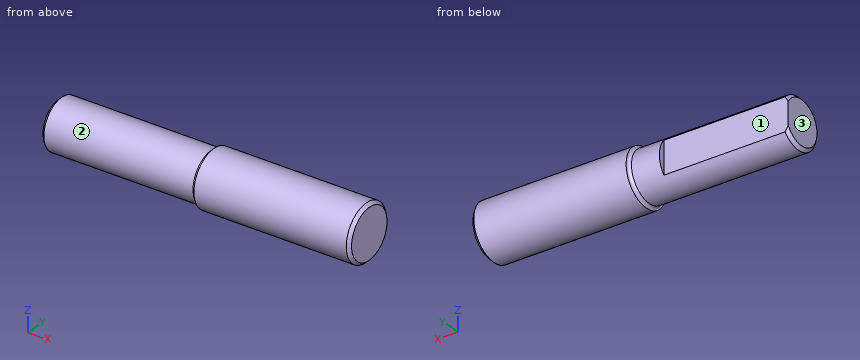
from build123d import *

# Parameters (mm, degrees)
CUT_EXTRUDE_1_DEPTH = 20


with BuildPart() as part:
    # 草图1 → 旋转1 (revolve)
    with BuildSketch(Plane.XY, mode=Mode.PRIVATE) as revolve_1_sk:
        with BuildLine():
            Line((25, 0), (25, 4))
            Line((25, 4), (24.5, 4.5))
            Line((24.5, 4.5), (0, 4.5))
            ThreePointArc((0, 4.5), (-0.146446609, 4.146446609), (-0.5, 4))
            Line((-0.5, 4), (-24.5, 4))
            Line((-24.5, 4), (-25, 3.5))
            Line((-25, 3.5), (-25, 0))
            Line((-25, 0), (25, 0))
        make_face()
    revolve(revolve_1_sk.sketch.rotate(Axis((-25, 0, 0), (1, 0, 0)), 180), axis=Axis((-25, 0, 0), (1, 0, 0)))

    # 草图2 → 切除-拉伸1 (cut)
    with BuildSketch(Plane.ZY.offset(25)):
        with BuildLine():
            Line((-2.645751311, 3), (2.645751311, 3))
            ThreePointArc((2.645751311, 3), (0, 4), (-2.645751311, 3))
        make_face()
    extrude(amount=-CUT_EXTRUDE_1_DEPTH, mode=Mode.SUBTRACT)


solid = part.part
Verification items for the finished model (mm, model axes). Face numbers are marked on the shaded views. A direction names the side the tool comes from. Give positions to 0.01 mm unless a question says otherwise; leave off trailing zeros. Loops run counter-clockwise (first coordinate to the right, second up) from the corner with the lowest first, then second, coordinate; pieces in that order, holes last.
1) Depth check by flat-ended pin: pin 1 Ø1 at (x, y) = (18, 1) entering from -Z; pin 2 Ø1 at (x, z) = (19, -2) entering from -Y. Enter the tip coordinate at first touch or a pass-through.
2) Sectioned sample at B-B, the plane y = 0. Enter the section's corners in (x, z).
3) Set-up check for the marked faces 1, 2 and 3: record each of +Z, -Z, +X, -X, +Y, -Y from which the full face is reachable in a straight line by a thin tool's end or side.
4) Sectioned sample at C-C, the plane x = -12.5. Enter the section's corners in (y, z).
5) Sectioned sample at A-A, the plane z = 0. Enter the section's corners in (x, y), then the cut area to 3 significant figures.
6) Sectioned sample at D-D, the plane x = 18. Enter the section's corners in (y, z).
7) Thickness scan on line 1 along Z through (x, y) = (-2, 3); line 2 along Y through (x, z) = (18, 2.5). Record the ranges inside material, lowest first.
Answers:
1. pin 1: stops at z = -4.47
1. pin 2: stops at y = -4.24
2. outline: (-25, -3.5) - (-24.5, -4) - (-0.5, -4) arc R0.5 cw to (0, -4.5) - (24.5, -4.5) - (25, -4) - (25, 4) - (24.5, 4.5) - (0, 4.5) arc R0.5 cw to (-0.5, 4) - (-24.5, 4) - (-25, 3.5) - close
3. face 1: +Z, -Z, -X, +Y
3. face 2: -X
3. face 3: +Z, -Z, -X, +Y, -Y
4. outline: (3, -2.65) - (3, 2.65) arc R4 ccw (long way) to start
5. outline: (-25, -3.5) - (-24.5, -4) - (-0.5, -4) arc R0.5 cw to (0, -4.5) - (24.5, -4.5) - (25, -4) - (25, 4) - (24.5, 4.5) - (0, 4.5) arc R0.5 cw to (-0.5, 4) - (-5, 4) - (-5, 3) - (-25, 3) - close
5. area: 405 mm2
6. outline: circle Ø9 at (0, 0)
7. line 1: z = -2.65 to 2.65
7. line 2: y = -3.74 to 3.74
